Source: CAD feature listing. Evaluate the final solid. Frame: model axes, mm. A direction names the side the tool comes from. Round coordinates to 2 decimals unless told otherwise and drop trailing zeros. Order: outer loops, then holes, each group sorted by start corner. A loop starts at its lowest first (then second) coordinate and runs counter-clockwise, first axis right, second up. Notation, with made-up numbers: (22.25, -17) - (41.25, -17) arc R21 cw to (41.25, -4) - close; hole circle Ø8 at (16, 54). An arc over 180 degrees is marked (long way). Put each result on its own line as item: value. Start each with the question number.
1) Section A-A on x = -38. Output: boundary loops of the cut face in (y, z), then the cut area to 3 significant figures.
2) Section B-B on z = 26.5. Output: boundary loops of the cut face in (x, y), then the cut area to 3 significant figures.
3) Line query: probe 1 along X at (y, z) = (48, 5.5); probe 2 along Y at (x, z) = (80, 25); probe 3 along Z at (x, y) = (4.5, -11). Output: solid intervals per line, ascending. Write a range as [from, to].
4) Access query for faces 1 (the face through (4, 45, 3)), 2 (the face through (127.853, 16.726, 1.521)). Directions: +Z, -Z, +X, -X, +Y, -Y. A direction counts if a zero-diameter tool reaches every point of the face in a straight line with its end or side. Return the directions, or none.
5) Contact query for flat-ended pins moving along their axis: P1, Ø3.5, axis at x = 3.5, y = 43, coming from the +Z side; P2, Ø4.5, axis at x = 123.99, y = 37.42, coming from the +Z side (1 decimal); P3, Ø8.5, axis at x = 79, y = 27, coming from the +Z side; P4, Ø4, axis at x = 44.5, y = 53, coming from the +Z side. Output: stop coordinate, or through.
6) Mould query, pull axis Y, two halves, no side actions, for faces 3 (the face through (40, 60, 2)), 4 (the face through (154.888, 68.775, 1.521)), 5 (the face through (44, 58, 22.7)). Classes: +Y half, -Y half, draft (parallel to the pull), parting line (faces both ways), or undercut.
```python
from build123d import *

# Parameters (mm, degrees)
SKETCH1_W           = 180
SKETCH1_H           = 78
SKETCH1_R           = 4
BOSS_EXTRUDE1_DEPTH = 3
SKETCH2_R           = 2.5
CUT_EXTRUDE1_DEPTH  = 3
SKETCH4_R           = 2.5
CUT_EXTRUDE3_DEPTH  = 10
SKETCH5_R           = 2.5
BOSS_EXTRUDE2_DEPTH = 3
SKETCH6_R           = 2.5
BOSS_EXTRUDE3_DEPTH = 3
SKETCH7_R           = 2.5
CUT_EXTRUDE4_DEPTH  = 179.975122888
SKETCH8_R           = 5.75
SKETCH8_R_2         = 3.8
BOSS_EXTRUDE4_DEPTH = 13.7
SKETCH9_R           = 5.75
SKETCH9_R_2         = 3.8
BOSS_EXTRUDE5_DEPTH = 7.7
SKETCH10_R          = 5.75
SKETCH10_R_2        = 3.8
BOSS_EXTRUDE6_DEPTH = 19.7
SKETCH11_R          = 5.75
SKETCH11_R_2        = 3.8
BOSS_EXTRUDE7_DEPTH = 25.7
CHAMFER1_SIZE       = 5
SKETCH12_R          = 5.5
SKETCH12_R_2        = 3.8
BOSS_EXTRUDE8_DEPTH = 31.7
CHAMFER2_SIZE       = 5
SKETCH13_R          = 2.5
CUT_EXTRUDE5_DEPTH  = 183.283253791


with BuildPart() as part:
    # Sketch1 → Boss-Extrude1 (new body)
    with BuildSketch(Plane.XY):
        with Locations((60, 21)):
            Rectangle(SKETCH1_W, SKETCH1_H)
        Circle(SKETCH1_R, mode=Mode.SUBTRACT)
    extrude(amount=BOSS_EXTRUDE1_DEPTH)

    # Sketch2 → Cut-Extrude1 (cut)
    with BuildSketch(Plane.XY.offset(3)):
        with Locations((1.379644584, 45.502149563)):
            Circle(SKETCH2_R)
        with Locations((30.30508702, 11.030149622)):
            Circle(SKETCH2_R)
        with Locations((45.55286784, 54.088554355)):
            Circle(SKETCH2_R)
        with Locations((80.524436105, 25.769136757)):
            Circle(SKETCH2_R)
        with Locations((123.991098288, 37.415993787)):
            Circle(SKETCH2_R)
        with Locations((130.350182866, 16.616365345)):
            Circle(SKETCH2_R)
    extrude(amount=-CUT_EXTRUDE1_DEPTH, mode=Mode.SUBTRACT)

    # Sketch4 → Cut-Extrude3 (cut)
    with BuildSketch(Plane.XY.offset(3)):
        with Locations((54, -12)):
            Circle(SKETCH4_R)
        with Locations((-19, -12)):
            Circle(SKETCH4_R)
        with Locations((116, -12)):
            Circle(SKETCH4_R)
    extrude(amount=-CUT_EXTRUDE3_DEPTH, mode=Mode.SUBTRACT)

    # Sketch5 → Boss-Extrude2 (add)
    # profile 1 of 2: a face of its own
    with BuildSketch(Plane.XY.offset(3)):
        with BuildLine():
            Line((116.068060007, 60), (116.068060007, 53.293456509))
            Line((116.068060007, 53.293456509), (63.931939993, 53.293456509))
            Line((63.931939993, 53.293456509), (63.931939993, 60))
            ThreePointArc((63.931939993, 60), (76.652430488, 63.648363172), (85.505506895, 73.48423987))
            ThreePointArc((85.505506895, 73.48423987), (90, 76.293456509), (94.494493105, 73.48423987))
            ThreePointArc((94.494493105, 73.48423987), (103.347569512, 63.648363172), (116.068060007, 60))
        make_face()
        with Locations((90, 71.293456509)):
            Circle(SKETCH5_R, mode=Mode.SUBTRACT)
    # profile 2 of 2: a face of its own
    with BuildSketch(Plane.XY.offset(3)):
        with BuildLine():
            Line((15.048465346, 60), (-9.629718418, 52.415464707))
            Line((-9.629718418, 52.415464707), (-30, 33.284639637))
            ThreePointArc((-30, 33.284639637), (-33.061352956, 51.208206171), (-41.898305085, 67.099537024))
            ThreePointArc((-41.898305085, 67.099537024), (-41.737026969, 73.552387313), (-35.347576733, 74.469018739))
            ThreePointArc((-35.347576733, 74.469018739), (-11.167529583, 63.688874665), (15.048465346, 60))
        make_face()
        with Locations((-38, 70.230546041)):
            Circle(SKETCH5_R, mode=Mode.SUBTRACT)
    extrude(amount=-BOSS_EXTRUDE2_DEPTH)

    # Sketch6 → Boss-Extrude3 (add)
    with BuildSketch(Plane.XY.offset(3)):
        with BuildLine():
            Line((103.71791688, 60), (150, 34.801241353))
            ThreePointArc((150, 34.801241353), (152.78836529, 51.929243873), (160.8654989, 67.28838981))
            ThreePointArc((160.8654989, 67.28838981), (160.554300014, 73.67838942), (154.213881277, 74.531636156))
            ThreePointArc((154.213881277, 74.531636156), (129.990577907, 63.705162892), (103.71791688, 60))
        make_face()
        with Locations((156.871563613, 70.296459112)):
            Circle(SKETCH6_R, mode=Mode.SUBTRACT)
    extrude(amount=-BOSS_EXTRUDE3_DEPTH)

    # Sketch7 → Cut-Extrude4 (cut, through all)
    with BuildSketch(Plane.XY.offset(3)):
        with Locations((11.891570779, -14.171822198)):
            Circle(SKETCH7_R)
        with Locations((-17.384313485, 6.327372652)):
            Circle(SKETCH7_R)
    extrude(amount=-CUT_EXTRUDE4_DEPTH, mode=Mode.SUBTRACT)

    # Sketch8 → Boss-Extrude4 (add)
    with BuildSketch(Plane.XY.offset(3)):
        with Locations(Location((1.379644584, 45.502149563, 0), (0, 0, 180))):
            Circle(SKETCH8_R)
        with Locations(Location((1.379644584, 45.502149563, 0), (0, 0, 180))):
            Circle(SKETCH8_R_2, mode=Mode.SUBTRACT)
    extrude(amount=BOSS_EXTRUDE4_DEPTH)

    # Sketch9 → Boss-Extrude5 (add)
    with BuildSketch(Plane.XY.offset(3)):
        with Locations(Location((30.30508702, 11.030149622, 0), (0, 0, 180))):
            Circle(SKETCH9_R)
        with Locations(Location((30.30508702, 11.030149622, 0), (0, 0, 180))):
            Circle(SKETCH9_R_2, mode=Mode.SUBTRACT)
    extrude(amount=BOSS_EXTRUDE5_DEPTH)

    # Sketch10 → Boss-Extrude6 (add)
    with BuildSketch(Plane.XY.offset(3)):
        with Locations(Location((45.55286784, 54.088554355, 0), (0, 0, 180))):
            Circle(SKETCH10_R)
        with Locations((45.55286784, 54.088554355)):
            Circle(SKETCH10_R_2, mode=Mode.SUBTRACT)
    extrude(amount=BOSS_EXTRUDE6_DEPTH)

    # Sketch11 → Boss-Extrude7 (add)
    with BuildSketch(Plane.XY.offset(3)):
        with Locations(Location((80.524436105, 25.769136757, 0), (0, 0, 180))):
            Circle(SKETCH11_R)
        with Locations(Location((80.524436105, 25.769136757, 0), (0, 0, 180))):
            Circle(SKETCH11_R_2, mode=Mode.SUBTRACT)
    extrude(amount=BOSS_EXTRUDE7_DEPTH)

    # Chamfer1
    # the kernel refuses this chamfer: 5 mm, written as the material it adds along each edge
    with BuildSketch(Plane(origin=(1.379644584, 45.502149563, 3), x_dir=(-1, 0, 0), z_dir=(0, 1, 0))) as chamfer1_piece_1:
        Polygon((5.75 + CHAMFER1_SIZE, 0), (5.75, CHAMFER1_SIZE), (5.75, 0), align=None)
    revolve(axis=Axis((1.379644584, 45.502149563, 3), (0, 0, 1)))
    with BuildSketch(Plane(origin=(30.30508702, 11.030149622, 3), x_dir=(-1, 0, 0), z_dir=(0, 1, 0))) as chamfer1_piece_2:
        Polygon((5.75 + CHAMFER1_SIZE, 0), (5.75, CHAMFER1_SIZE), (5.75, 0), align=None)
    revolve(axis=Axis((30.30508702, 11.030149622, 3), (0, 0, 1)))
    with BuildSketch(Plane(origin=(45.55286784, 54.088554355, 3), x_dir=(-1, 0, 0), z_dir=(0, 1, 0))) as chamfer1_piece_3_section:
        Polygon((5.75 + CHAMFER1_SIZE, 0), (5.75, CHAMFER1_SIZE), (5.75, 0), align=None)
    chamfer1_piece_3 = revolve(axis=Axis((45.55286784, 54.088554355, 3), (0, 0, 1)), mode=Mode.PRIVATE)
    chamfer1_piece_3 = split(chamfer1_piece_3, bisect_by=Plane(origin=(53.746055157, 60, 5.443187317), z_dir=(0, -1, 0)), keep=Keep.TOP, mode=Mode.PRIVATE)
    add(chamfer1_piece_3)
    with BuildSketch(Plane(origin=(80.524436105, 25.769136757, 3), x_dir=(-1, 0, 0), z_dir=(0, 1, 0))) as chamfer1_piece_4:
        Polygon((5.75 + CHAMFER1_SIZE, 0), (5.75, CHAMFER1_SIZE), (5.75, 0), align=None)
    revolve(axis=Axis((80.524436105, 25.769136757, 3), (0, 0, 1)))

    # Sketch12 → Boss-Extrude8 (add)
    with BuildSketch(Plane.XY.offset(3)):
        with Locations(Location((123.991098288, 37.415993787, 0), (0, 0, 180))):
            Circle(SKETCH12_R)
        with Locations((123.991098288, 37.415993787)):
            Circle(SKETCH12_R_2, mode=Mode.SUBTRACT)
    extrude(amount=BOSS_EXTRUDE8_DEPTH)

    # Chamfer2
    chamfer2_edges = [part.edges().sort_by_distance(p)[0] for p in [
        (129.491098288, 37.415993787, 3),
    ]]
    chamfer(chamfer2_edges, length=CHAMFER2_SIZE)

    # Sketch13 → Cut-Extrude5 (cut, through all)
    with BuildSketch(Plane(origin=(0, 0, 0), x_dir=(-1, 0, 0), z_dir=(0, 0, -1))):
        with Locations((-16.2, -2)):
            Circle(SKETCH13_R)
        with Locations((16.2, -2)):
            Circle(SKETCH13_R)
    extrude(amount=-CUT_EXTRUDE5_DEPTH, mode=Mode.SUBTRACT)


solid = part.part
```
Answer sheet:
1. outline: (61.57, 0) - (67.73, 0) - (67.73, 3) - (61.57, 3) - close; (72.73, 0) - (75.23, 0) - (75.23, 3) - (72.73, 3) - close
1. area: 26.0 mm^2
2. outline: circle Ø11.5 at (80.52, 25.77); circle Ø11 at (123.99, 37.42); hole circle Ø7.6 at (80.52, 25.77); hole circle Ø7.6 at (123.99, 37.42)
2. area: 108 mm^2
3. probe 1: [-6.48, -1.48], [4.24, 9.24], [39.99, 51.12]
3. probe 2: [20.04, 22.01], [29.53, 31.5]
3. probe 3: [0, 3]
4. face 1: +Z
4. face 2: +Z, -Z
5. P1: z = 16.7
5. P2: through
5. P3: z = 28.7
5. P4: z = 3
6. face 3: +Y half
6. face 4: undercut
6. face 5: draft
